```python
from build123d import *

# Parameters (mm, degrees)
SKETCH1_W           = 12.2
SKETCH1_H           = 22.6
BOSS_EXTRUDE1_DEPTH = 24
BOSS_EXTRUDE2_DEPTH = 2.5
BOSS_EXTRUDE3_DEPTH = 4.75


with BuildPart() as part:
    # Sketch1 → Boss-Extrude1 (new body)
    with BuildSketch(Plane(origin=(0, 0, 0), x_dir=(1, 0, 0), z_dir=(0, 1, 0))):
        with Locations((6.1, 11.3)):
            Rectangle(SKETCH1_W, SKETCH1_H)
    extrude(amount=BOSS_EXTRUDE1_DEPTH)

    # Sketch2 → Boss-Extrude2 (add)
    with BuildSketch(Plane(origin=(0, 19.5, 0), x_dir=(1, 0, 0), z_dir=(0, 1, 0))):
        with BuildLine():
            Line((0, 22.6), (12.2, 22.6))
            Line((12.2, 22.6), (12.2, 28.1))
            Line((12.2, 28.1), (6.6, 28.1))
            Line((6.6, 28.1), (6.6, 27.55399362))
            ThreePointArc((6.6, 27.55399362), (6.1, 24.95), (5.6, 27.55399362))
            Line((5.6, 27.55399362), (5.6, 28.1))
            Line((5.6, 28.1), (0, 28.1))
            Line((0, 28.1), (0, 22.6))
        make_face()
    boss_extrude2 = extrude(amount=-BOSS_EXTRUDE2_DEPTH)

    # Mirror1: Boss-Extrude2 across plane
    add(boss_extrude2.mirror(Plane.XY.offset(-11.3)))

    # Sketch6 → Boss-Extrude3 (add)
    with BuildSketch(Plane(origin=(0, 24, 0), x_dir=(1, 0, 0), z_dir=(0, 1, 0))):
        with BuildLine():
            ThreePointArc((8.704115376, 11.616210937), (6.1, 0), (3.495884624, 11.616210937))
            ThreePointArc((3.495884624, 11.616210937), (6.1, 15.25), (8.704115376, 11.616210937))
        make_face()
    extrude(amount=BOSS_EXTRUDE3_DEPTH)


solid = part.part
```
CAD build for the part. Positions are in the model's coordinates, mm. A direction names the side the tool comes from. Round coordinates to 2 decimals unless told otherwise and drop trailing zeros. Write each loop counter-clockwise with the first axis right and the second up, starting at its lowest first coordinate (ties: lowest second). Pieces come first, ordered by that corner, then holes. Notation, with made-up numbers: (55.5, 80.25) - (96.5, 80.25) arc R16 cw to (96.5, 96.25) - close; hole circle Ø6 at (64, 1). An arc over 180 degrees is marked (long way). Write item = value, one per line. Start each with the question number.
Q1. Band-saw the part on C-C (x = 2). Give the cut face in (y, z).
Q2. Probe L1, parallel to X at y = 18.8, z = -26.3; L2, parallel to Y at x = 10.25, z = -14; L3, parallel to Z at x = 1.5, y = 23. List the from-to ranges inside material, lowest first. Write a range as from..to.
Q3. Band-saw the part on B-B (z = -12.5). Give the cut face in (x, y), then the cut area to 3 significant figures.
Q4. Drop flat-ended pins along their axis: pin 1 (3 mm diameter, centred on x = 4.5, z = -26, fed in from +Y); pin 2 (5 mm diameter, centred on x = 3, y = 20.5, fed in from +Z); pin 3 (4.5 mm diameter, centred on x = 9, z = -25, fed in from -Y); pin 4 (4 mm diameter, centred on x = 4.5, y = 22, fed in from -Z). Give the stop position or say it passes through.
Q5. Band-saw the part on D-D (y = 24.75). Give the cut face in (x, z).
Q6. Which spindle directions (+Z, -Z, +X, -X, +Y, -Y) get a long thin tool onto all of the face, cutting with end or side? Do faces 5 (the flat face through (6, 8, 0)), 6 (the flat face through (6, 22, 0)), 7 (the cylindrical face through (6, 26, 0)), 8 (the flat face through (6, 8, -22.6)). Say none if no direction does.
Q7. Mould opens along Z. For faces 1 (the flat face through (9, 18, 5.5)), 2 (the flat face through (9, 18, -28.1)), 3 (the flat face through (6, 28.75, -8)), 4 (the cylindrical face through (6.03, 26.34, -15.25)) say: pulls with the +Z half, pulls with the -Z half, needs draft (parallel to the pull), parting line crosses it, or undercut.
Q8. Band-saw the part on A-A (z = -26.3). Give the cut face in (x, y), then the cut area to 4 significant figures.
Answers below:
q1.outline = (0, -22.6) - (17, -22.6) - (17, -28.1) - (19.5, -28.1) - (19.5, -22.6) - (24, -22.6) - (24, -10.62) - (28.75, -10.62) - (28.75, -1.58) - (24, -1.58) - (24, 0) - (19.5, 0) - (19.5, 5.5) - (17, 5.5) - (17, 0) - (0, 0) - close
q2.L1 = 0..4.75, 7.45..12.2
q2.L2 = 0..24
q2.L3 = -22.6..0
q3.outline = (0, 0) - (12.2, 0) - (12.2, 24) - (8.85, 24) - (8.85, 28.75) - (3.35, 28.75) - (3.35, 24) - (0, 24) - close
q3.area = 319 mm2
q4.pin_1 = 19.5
q4.pin_2 = 5.5
q4.pin_3 = 17
q4.pin_4 = -22.6
q5.outline = (3.5, -11.62) arc R2.75 ccw (long way) to (8.7, -11.62) arc R6.1 ccw (long way) to start
q6.face_5 = +Z, +X, -X, -Y
q6.face_6 = +Z, +X, -X, +Y
q6.face_7 = +Y
q6.face_8 = -Z, +X, -X, -Y
q7.face_1 = pulls with the +Z half
q7.face_2 = pulls with the -Z half
q7.face_3 = needs draft
q7.face_4 = undercut
q8.outline = (0, 17) - (4.75, 17) - (4.75, 19.5) - (0, 19.5) - close; (7.45, 17) - (12.2, 17) - (12.2, 19.5) - (7.45, 19.5) - close
q8.area = 23.75 mm2
